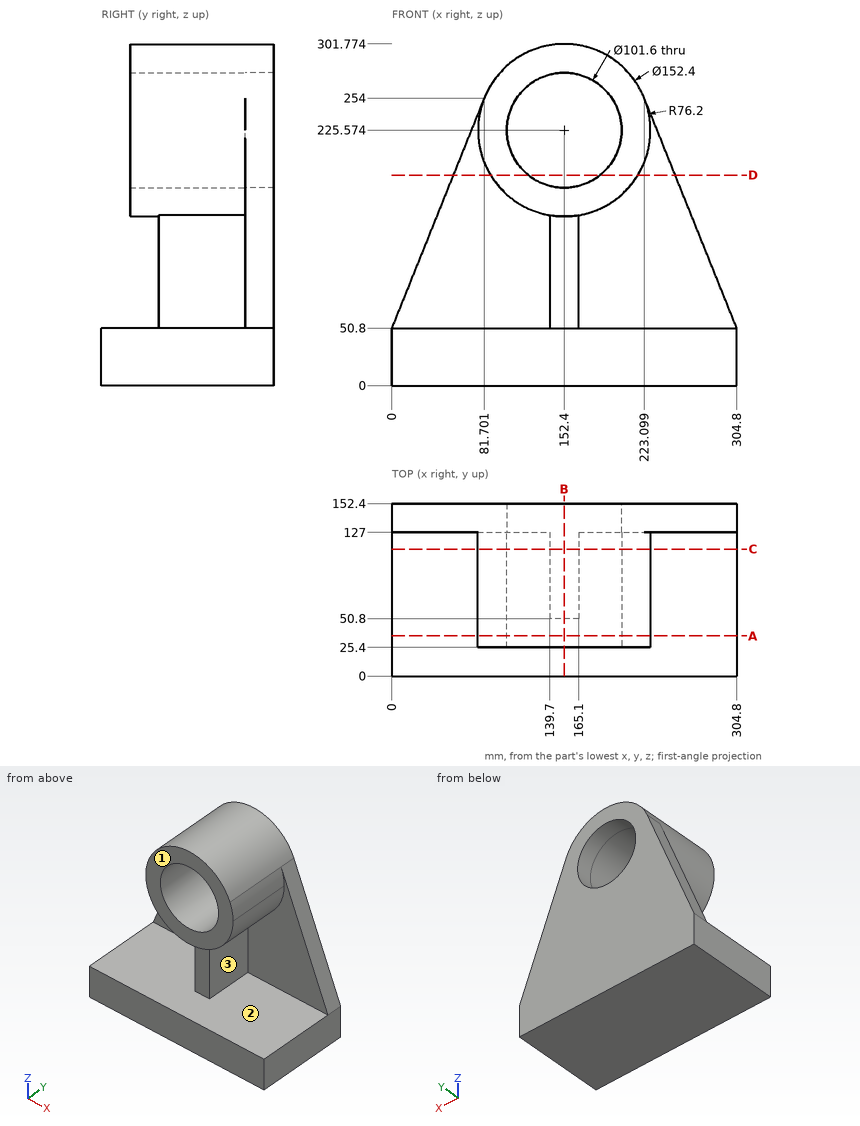
Can you work these out from the drawing? Everything is in mm from the part's minimum corner. A direction names the side the tool comes from. Give positions to 0.01 mm unless a question says otherwise; leave off trailing zeros. Loops run counter-clockwise (first coordinate to the right, second up) from the corner with the lowest first, then second, coordinate; pieces in that order, holes last. Notation, with made-up numbers: (15, 14.25) - (64, 14.25) arc R20 cw to (64, 22.25) - close; hole circle Ø5 at (-0.75, 36.25). An arc over 180 degrees is marked (long way). Answer as a JSON object with one key per item and string values.
Q1. Will these pins go through, and if not, where does the flat tip stop? P1, Ø23, axis at y = 100.5, z = 114.5, coming from the -X side; P2, Ø7.5, axis at x = 149, z = 96.5, coming from the -Y side; P3, Ø1, axis at y = 120, z = 271, coming from the -X side; P4, Ø8, axis at x = 265, z = 161, coming from the -Y side.
Geometry says:
{"P1": "x = 139.7", "P2": "y = 50.8", "P3": "x = 90.85", "P4": "through"}
Q2. Imagine slicing it at A-A on y = 35.5. Write out the boundary of the cut face in (x, z), plus the area to 3 significant figures.
Geometry says:
{"outline": "(0, 0) - (304.8, 0) - (304.8, 50.8) - (0, 50.8) - close; circle Ø152.4 at (152.4, 225.57); hole circle Ø101.6 at (152.4, 225.57)", "area": "25,600 mm²"}
Q3. Which directions (+Z, -Z, +X, -X, +Y, -Y) give clear straight access to the entire face, cutting with the end or side of a thin tool? Please do the marked faces 1, 2 and 3.
Geometry says:
{"face 1": "+Z, +X, -X, -Y", "face 2": "-Y", "face 3": "+X, -Y"}
Q4. Imagine slicing it at B-B on x = 152.4. Write out the boundary of the cut face in (y, z), plus the area to 3 significant figures.
Geometry says:
{"outline": "(0, 0) - (152.4, 0) - (152.4, 174.77) - (25.4, 174.77) - (25.4, 149.37) - (50.8, 149.37) - (50.8, 50.8) - (0, 50.8) - close; (25.4, 276.37) - (152.4, 276.37) - (152.4, 301.77) - (25.4, 301.77) - close", "area": "24,200 mm²"}
Q5. Imagine slicing it at C-C on y = 112. Write out the boundary of the cut face in (x, z).
Geometry says:
{"outline": "(0, 0) - (304.8, 0) - (304.8, 50.8) - (165.1, 50.8) - (165.1, 150.44) arc R76.2 ccw (long way) to (139.7, 150.44) - (139.7, 50.8) - (0, 50.8) - close; hole circle Ø101.6 at (152.4, 225.57)"}
Q6. Imagine slicing it at D-D on z = 186. Write out the boundary of the cut face in (x, y).
Geometry says:
{"outline": "(54.36, 127) - (87.28, 127) - (87.28, 25.4) - (120.55, 25.4) - (120.55, 152.4) - (54.36, 152.4) - close; (184.25, 25.4) - (217.52, 25.4) - (217.52, 127) - (250.44, 127) - (250.44, 152.4) - (184.25, 152.4) - close"}
Q7. If I drill on L1, parallel to Z at x = 152, y = 135 (1 decimal); L2, parallel to Y at x = 258.5, z = 163; L3, parallel to Z at x = 53, y = 44, over which ranges is the centre line in solid material (lowest first)?
Geometry says:
{"L1": "0 to 174.8, 276.4 to 301.8", "L2": "127 to 152.4", "L3": "0 to 50.8"}
